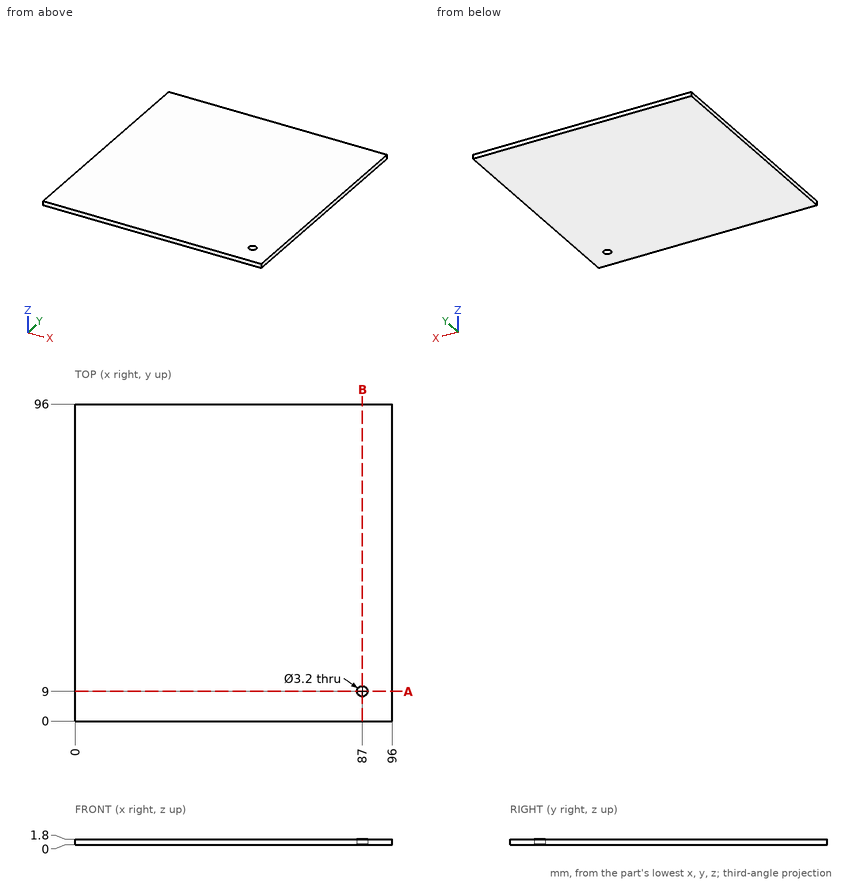
Study the drawing (mm; zero at the part's minimum x, y, z) and answer. Give positions to 0.01 mm unless a question says otherwise; leave off trailing zeros. Loops run counter-clockwise (first coordinate to the right, second up) from the corner with the lowest first, then second, coordinate; pieces in that order, holes last. Notation, with made-up numbers: (85, -39) - (142, -39) arc R26 cw to (142, -5) - close; hole circle Ø8 at (22, 54). An arc over 180 degrees is marked (long way). Answer as CSV lines item,"result". Start each with the question number.
1) This flat-tipped pin is pushed along its axis until it touches: pin 1 Ø1.9 at (x, y) = (87, 9) entering from -Z. Where does it stop, or does it pass through?
2) Find section B-B (x = 87). Write down the section's boundary in (y, z), then the cut area to 3 significant figures.
3) A straight line is drawn through the part: L1, parallel to Y at x = 87, z = 0.9. Find the intervals that lie inside material, in ascending order. Write a range as from..to.
4) Find section A-A (y = 9). Write down the section's boundary in (x, z).
Findings below:
1,pin 1,"through"
2,outline,"(0, 0) - (7.4, 0) - (7.4, 1.8) - (0, 1.8) - close; (10.6, 0) - (96, 0) - (96, 1.8) - (10.6, 1.8) - close"
2,area,"167 mm^2"
3,L1,"0..7.4, 10.6..96"
4,outline,"(0, 0) - (85.4, 0) - (85.4, 1.8) - (0, 1.8) - close; (88.6, 0) - (96, 0) - (96, 1.8) - (88.6, 1.8) - close"
